Autodesk Inventor part; units mm, degrees
ref_plane "YZ Plane" through (0, 0, 0) normal (1, 0, 0) x (0, 1, 0)
ref_plane "XZ Plane" through (0, 0, 0) normal (0, 1, 0) x (-1, 0, 0)
ref_plane "XY Plane" through (0, 0, 0) normal (0, 0, 1) x (1, 0, 0)
sketch "Sketch1" plane through (0, 0, 0) normal (0, 0, 1) x (1, 0, 0)
  line L0 (-23.55, 23.55) -> (23.55, 23.55) construction
  line L1 (23.55, 23.55) -> (23.55, -23.55) construction
  line L2 (23.55, -23.55) -> (-23.55, -23.55) construction
  line L3 (-23.55, -23.55) -> (-23.55, 23.55) construction
  line L4 (0, 23.55) -> (0, -23.55) construction
  line L5 (-23.55, 0) -> (23.55, 0) construction
  circle A0 centre (-23.55, 23.55) radius 2.75
  circle A1 centre (23.55, 23.55) radius 2.75
  circle A2 centre (-23.55, -23.55) radius 2.75
  circle A3 centre (23.55, -23.55) radius 2.75
  circle A4 centre (0, 0) radius 20
  line L6 (-28.2, 28.2) -> (28.2, 28.2) construction
  line L7 (28.2, 28.2) -> (28.2, -28.2) construction
  line L8 (28.2, -28.2) -> (-28.2, -28.2) construction
  line L9 (-28.2, -28.2) -> (-28.2, 28.2) construction
  line L10 (-28.2, 0) -> (28.2, 0) construction
  line L11 (0, -28.2) -> (0, 28.2) construction
  line L12 (-60, 21.2) -> (-32, 21.2) construction
  line L13 (-32, 21.2) -> (-32, -25.8) construction
  line L14 (-32, -25.8) -> (-60, -25.8) construction
  line L15 (-60, -25.8) -> (-60, 21.2) construction
  line L16 (-46, 21.2) -> (-46, -25.8) construction
  line L17 (-60, -2.3) -> (-32, -2.3) construction
  circle A5 centre (-46, 15.7) radius 2.75
  circle A6 centre (-46, -20.3) radius 2.75
  line L18 (60, 21.2) -> (32, 21.2) construction
  line L19 (32, 21.2) -> (32, -25.8) construction
  line L20 (32, -25.8) -> (60, -25.8) construction
  line L21 (60, -25.8) -> (60, 21.2) construction
  line L22 (46, 21.2) -> (46, -25.8) construction
  line L23 (60, -2.3) -> (32, -2.3) construction
  circle A7 centre (46, 15.7) radius 2.75
  circle A8 centre (46, -20.3) radius 2.75
  line L24 (-82, 43.2) -> (82, 43.2)
  line L25 (82, 43.2) -> (82, -43.2)
  line L26 (82, -43.2) -> (-82, -43.2)
  line L27 (-82, -43.2) -> (-82, 43.2)
  point P0 (0, 0)
  dimension "d0" = 47.1
  dimension "d1" = 47.1
  dimension "d2" = 5.5
  dimension "d4" = 40
  dimension "d5" = 56.4
  dimension "d6" = 56.4
  dimension "d9" = 46
  dimension "d10" = 47
  dimension "d11" = 28
  dimension "d12" = 5.5
  dimension "d13" = 36
  dimension "d14" = 22
  dimension "d15" = 15
  dimension "d18" = 2.3
extrude "Extrusion1" add sketch "Sketch1" along normal blind 10
sketch "Sketch2" plane through (0, 0, 0) normal (0, 0, -1) x (-1, 0, 0)
  line L0 (32.5, -32.5) -> (-32.5, -32.5)
  line L1 (-32.5, -32.5) -> (-32.5, 32.5)
  line L2 (-32.5, 32.5) -> (32.5, 32.5)
  line L3 (32.5, 32.5) -> (32.5, -32.5)
  line L4 (0, 32.5) -> (0, -32.5) construction
  line L5 (-32.5, 0) -> (32.5, 0) construction
  line L6 (-82, -43.2) -> (-82, 43.2)
  line L7 (82, -43.2) -> (-82, -43.2)
  line L8 (-82, 43.2) -> (82, 43.2)
  line L9 (82, 43.2) -> (82, -43.2)
  line L10 (82, -43.2) -> (-82, -43.2)
  line L11 (-82, -43.2) -> (-82, 43.2)
  point P0 (0, 0)
  point P1 (0, 0)
  dimension "d19" = 65
  dimension "d20" = 65
extrude "Extrusion2" add sketch "Sketch2" along normal blind 90
sketch "Sketch3" plane through (0, 0, 0) normal (0, 0, -1) x (-1, 0, 0)
  line L0 (32.5, -32.5) -> (32.5, 32.5)
  line L1 (32.5, 32.5) -> (-32.5, 32.5)
  line L2 (-32.5, 32.5) -> (-32.5, -32.5)
  line L3 (-32.5, -32.5) -> (32.5, -32.5)
  circle A0 centre (23.55, 23.55) radius 2.75
  circle A1 centre (-23.55, 23.55) radius 2.75
  circle A2 centre (23.55, -23.55) radius 2.75
  circle A3 centre (-23.55, -23.55) radius 2.75
  circle A4 centre (0, 0) radius 20
extrude "Extrusion3" add sketch "Sketch3" along normal blind 10
sketch "Sketch4" plane through (-82, -43.2, 10) normal (-1, 0, 0) x (0, 0, 1)
  line L0 (0, 0) -> (-100, 0)
  line L1 (0, 86.4) -> (0, 0)
  line L2 (-100, 86.4) -> (0, 86.4)
  line L3 (-100, 0) -> (-100, 86.4)
  point P0 (-10, 43.2)
extrude "Extrusion4" add sketch "Sketch4" along normal blind 10
sketch "Sketch5" plane through (82, -43.2, -90) normal (0, -1, 0) x (1, 0, 0)
  line L0 (-174, 0) -> (-174, 100) construction
  line L1 (-174, 50) -> (0, 50) construction
  line L2 (0, 0) -> (0, 100) construction
  line L3 (0, 100) -> (-174, 100) construction
  line L4 (-87, 100) -> (-87, 0) construction
  line L5 (0, 0) -> (-174, 0) construction
  circle A0 centre (-87, 50) radius 27.305
  point P0 (-82, 90)
  dimension "d27" = 54.61
extrude "Extrusion5" add sketch "Sketch5" along normal blind 50
sketch "Sketch6" plane through (-92, -43.2, 10) normal (-1, 0, 0) x (0, 0, 1)
  line L0 (-100, 75.7) -> (-100, 10.7) construction
  line L1 (-100, 43.2) -> (0, 43.2) construction
  line L2 (0, 0) -> (0, 86.4) construction
  line L3 (-100, 86.4) -> (0, 86.4) construction
  line L4 (-50, 86.4) -> (-50, 0) construction
  line L5 (-100, 0) -> (0, 0) construction
  circle A0 centre (-50, 43.2) radius 27.305
  point P0 (-10, 43.2)
  dimension "d30" = 54.61
extrude "Extrusion6" add sketch "Sketch6" along normal blind 50
sketch "Sketch7" plane through (-142, 0, -40) normal (-1, 0, 0) x (0, 0, 1)
  circle A0 centre (0, 0) radius 27.305
  circle A1 centre (0, 0) radius 10
  point P0 (40, 0)
  dimension "d33" = 20
extrude "Extrusion7" cut sketch "Sketch7" against normal up to surface (109.5 mm away) contours A1
sketch "Sketch8" plane through (82, 43.2, 10) normal (0, 1, 0) x (1, 0, 0)
  line L0 (-174, 100) -> (-174, 0) construction
  line L1 (-174, 0) -> (-154, 0) construction
  line L2 (-154, 0) -> (-154, 10) construction
  line L3 (-154, 10) -> (-174, 10) construction
  line L4 (-174, 10) -> (-174, 0) construction
  line L5 (0, 0) -> (-174, 0) construction
  line L6 (-154, 10) -> (-139, 10) construction
  line L7 (-139, 10) -> (-139, 0) construction
  line L8 (-139, 0) -> (-154, 0) construction
  line L9 (-154, 0) -> (-154, 10) construction
  circle A0 centre (-139, 10) radius 2.5
  circle A1 centre (-154, 10) radius 2.5
  point P0 (-82, 10)
  dimension "d36" = 20
  dimension "d37" = 10
  dimension "d38" = 15
  dimension "d39" = 5
  dimension "d40" = 5
extrude "Extrusion8" cut sketch "Sketch8" against normal blind 6
sketch "Sketch9" plane through (82, 43.2, 10) normal (0, 1, 0) x (1, 0, 0)
  line L0 (-174, 0) -> (-174, 100) construction
  line L1 (-174, 50) -> (0, 50) construction
  line L2 (0, 100) -> (0, 0) construction
  circle A0 centre (-139, 10) radius 2.5 construction
  circle A1 centre (-154, 10) radius 2.5 construction
  line L3 (-139, 10) -> (-154, 10) construction
  line L4 (-146.5, 10) -> (-146.5, 50) construction
  circle A2 centre (-146.5, 50) radius 10
  point P0 (-82, 10)
  dimension "d43" = 20
extrude "Extrusion9" cut sketch "Sketch9" against normal blind 43.2
properties part number "driver_L"
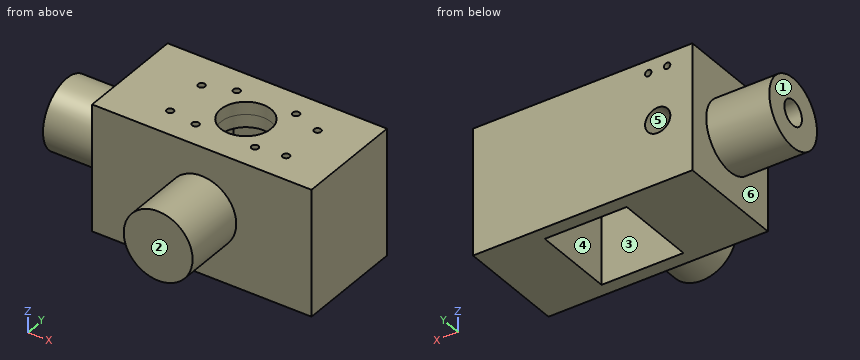
Input: part model. Units: mm. Frame: model coordinates. Face numbers are marked on the shaded views. A direction names the side the tool comes from. Coordinates: 2 decimals unless noted, no trailing zeros. Loops run counter-clockwise (first coordinate to the right, second up) from the corner with the lowest first, then second, coordinate; pieces in that order, holes last. Notation, with made-up numbers: (-5.5, 67.25) - (33.5, 67.25) arc R18 cw to (33.5, 100.25) - close; hole circle Ø2 at (71.25, -17). An arc over 180 degrees is marked (long way). Answer in a Markdown table with one row per item. Add a question column.
Item 1: Section query A-A on z = -78.5. Return the cut outline in (x, y).
Item 2: Section query D-D on x = -13.5. Return the cut outline in (y, z), then the cut area to 3 significant figures.
Item 3: Line query: line 1 along Y through (x, z) = (-46, 5.5); line 2 along X through (y, z) = (-23.55, -1.75); line 3 along X through (y, z) = (-23, -3). Output: solid intervals per line, ascending. Write a range as [from, to].
Item 4: Section query C-C on z = -40. Return the cut outline in (x, y) (3 decimals).
Item 5: Mould query, pull axis X, two halves, no side actions, for the marked faces 1, 2 and 3. Classes: released by +X, released by -X, zero draft, split by the parting line, or undercut.
Item 6: Access query for the marked faces 4, 5 and 6. Directions: +Z, -Z, +X, -X, +Y, -Y. A direction counts if a zero-diameter tool reaches every point of the face in a straight line with its end or side. Return the directions, or none.
Item 7: Section query B-B on x = -64.5. Return the cut outline in (y, z).
Item 8: Contact query for flat-ended pins moving along their axis: P1, Ø4.5, axis at x = 45.5, y = 16, coming from the +Z side; P2, Ø10, axis at x = 43, z = -62, coming from the -Y side; P3, Ø2, axis at y = -3, z = -44.5, coming from the -X side; P4, Ø7, axis at x = -23.55, y = 23.55, coming from the -Z side. Output: stop coordinate, or through.
Recorded:
| question | item | result |
|---|---|---|
| 1 | outline | (-92, -43.2) - (82, -43.2) - (82, 43.2) - (-92, 43.2) - close; hole (-32.5, -32.5) - (32.5, -32.5) - (32.5, 32.5) - (-32.5, 32.5) - close |
| 2 | outline | (-93.2, -65.95) - (-43.2, -65.95) - (-43.2, -90) - (-32.5, -90) - (-32.5, -10) - (-14.76, -10) - (-14.76, 10) - (-43.2, 10) - (-43.2, -14.05) - (-93.2, -14.05) - close; (14.76, -10) - (32.5, -10) - (32.5, -90) - (43.2, -90) - (43.2, 10) - (14.76, 10) - close |
| 2 | area | 5,440 mm^2 |
| 3 | line 1 | [-43.2, -23.05], [-17.55, 12.95], [18.45, 43.2] |
| 3 | line 2 | [-92, -26.3], [-20.8, 20.8], [26.3, 82] |
| 3 | line 3 | [-92, -26.24], [-20.86, 20.86], [26.24, 82] |
| 4 | outline | (-142, -27.305) - (-92, -27.305) - (-92, -43.2) - (-32.305, -43.2) - (-32.305, -93.2) - (22.305, -93.2) - (22.305, -43.2) - (82, -43.2) - (82, 43.2) - (-54.5, 43.2) - (-54.5, 10) - (-32.5, 10) - (-32.5, 32.5) - (32.5, 32.5) - (32.5, -32.5) - (-32.5, -32.5) - (-32.5, -10) - (-142, -10) - close; (-142, 10) - (-74.5, 10) - (-74.5, 43.2) - (-92, 43.2) - (-92, 27.305) - (-142, 27.305) - close |
| 5 | face 1 | released by -X |
| 5 | face 2 | zero draft |
| 5 | face 3 | undercut |
| 6 | face 4 | -Z |
| 6 | face 5 | +Y |
| 6 | face 6 | -X |
| 7 | outline | (-43.2, -90) - (43.2, -90) - (43.2, -50) - (0, -50) arc R10 cw to (0, -30) - (43.2, -30) - (43.2, 10) - (-43.2, 10) - close |
| 8 | P1 | z = 10 |
| 8 | P2 | y = -43.2 |
| 8 | P3 | x = 32.5 |
| 8 | P4 | z = -10 |
